Check sheet for the modelled part. Datum: model origin and axes. Units: mm. A direction names the side the tool comes from. Round coordinates to 2 decimals unless told otherwise and drop trailing zeros. Loops run counter-clockwise (first coordinate to the right, second up) from the corner with the lowest first, then second, coordinate; pieces in that order, holes last. Notation, with made-up numbers: (61, 78.5) -> (82, 78.5) arc R8 ccw to (82, 82.5) -> close; hole circle Ø9 at (18, 64.5). An arc over 180 degrees is marked (long way). One line per question, with ' | ' between items.
```python
from build123d import *

# Parameters (mm, degrees)
SKETCH2_R = 3


with BuildPart() as part:
    # Sweep3: sweep along a path in Sketch1
    with BuildLine(Plane.XY) as sweep3_path:
        Line((-58.210678119, 50), (-33.210678119, 50))
        Line((-33.210678119, 50), (-12.5, 0))
        Line((-12.5, 0), (12.5, 0))
        Line((12.5, 0), (33.210678119, 50))
        Line((33.210678119, 50), (58.210678119, 50))
    # Sketch2 → Sweep3 (sweep)
    with BuildSketch(Plane(origin=(49, 0, 0), x_dir=(0, 0, -1), z_dir=(1, 0, 0))):
        with Locations((0, 50)):
            Circle(SKETCH2_R)
    sweep(path=sweep3_path.line, transition=Transition.RIGHT)


solid = part.part
```
(1) Sectioned sample at B-B, the plane x = -8. Record the cut outline in (y, z).
Answer:
outline: circle Ø6 at (0, 0)
(2) Scan lines: probe 1 along X at (y, z) = (46, -2); probe 2 along X at (y, z) = (15.5, -2); probe 3 along Z at (x, y) = (-39.5, 48). Record each from-to range of solid material in increasing order.
Answer:
probe 1: x = -33.97 to -29.13, 29.13 to 33.97 | probe 2: x = -21.34 to -16.5, 16.5 to 21.34 | probe 3: z = -2.24 to 2.24
(3) Set-up check for faces 1 (the face through (0.2, -2.93, 0.65)), 2 (the face through (58.211, 50, 0)), 3 (the face through (-45, 53, 0)): record each of +Z, -Z, +X, -X, +Y, -Y from which the full face is reachable in a straight line by a thin tool's end or side.
Answer:
face 1: none | face 2: +Z, -Z, +X, +Y, -Y | face 3: -X
(4) Go/stop test with flat-tipped pins: pin 1 (1 mm diameter, centred on y = 7.5, z = -0.5, fed in from -X); pin 2 (10 mm diameter, centred on x = 12, y = 16, fed in from -Z); pin 3 (2 mm diameter, centred on x = 44.5, z = 1.5, fed in from -Y). Record where each tip stops, or that it passes through.
Answer:
pin 1: stops at x = -19.03 | pin 2: stops at z = -2.55 | pin 3: stops at y = 47.04
(5) Mould release check, pull along X, two halves, no side actions. Record for faces 4 (the face through (-58.211, 50, 0)), 5 (the face through (20.67, 26.34, -1.61)), 6 (the face through (45, 53, 0)): +X half, -X half, draft (parallel to the pull), parting line (faces both ways), or undercut.
Answer:
face 4: -X half | face 5: undercut | face 6: draft
(6) Sectioned sample at A-A, the plane z = 0. Record the cut outline in (x, y).
Answer:
outline: (-58.21, 47) -> (-35.22, 47) -> (-14.5, -3) -> (14.5, -3) -> (35.22, 47) -> (58.21, 47) -> (58.21, 53) -> (31.21, 53) -> (10.5, 3) -> (-10.5, 3) -> (-31.21, 53) -> (-58.21, 53) -> close
